from build123d import *

# Parameters (mm, degrees)
SKETCH1_R           = 6
BOSS_EXTRUDE1_DEPTH = 6


with BuildPart() as part:
    # Sketch1 → Boss-Extrude1 (new body, symmetric)
    with BuildSketch(Plane(origin=(0, 0, 0), x_dir=(1, 0, 0), z_dir=(0, 1, 0))):
        Polygon((15.011106999, 0), (7.505553499, 13), (-7.505553499, 13), (-15.011106999, 0), (-7.505553499, -13), (7.505553499, -13), align=None)
        Circle(SKETCH1_R, mode=Mode.SUBTRACT)
    extrude(amount=BOSS_EXTRUDE1_DEPTH, both=True)

    # Sketch3 → Cut-Revolve1 (revolve, cut)
    with BuildSketch(Plane.XY):
        with BuildLine():
            Line((10.011106999, 6), (15.011106999, 6))
            Line((15.011106999, 6), (15.011106999, 1))
            ThreePointArc((15.011106999, 1), (13.546640905, 4.535533906), (10.011106999, 6))
        make_face()
    cut_revolve1 = revolve(axis=Axis((0, 1.164773658, 0), (0, 1, 0)), mode=Mode.SUBTRACT)

    # Mirror1: Cut-Revolve1 across plane
    add(cut_revolve1.mirror(Plane.ZX), mode=Mode.SUBTRACT)


solid = part.part
Geometry: final body of the model. Coordinates: model frame, mm. Round coordinates to 2 decimals unless told otherwise and drop trailing zeros. Loops run counter-clockwise (first coordinate to the right, second up) from the corner with the lowest first, then second, coordinate; pieces in that order, holes last.
Q1. Material intervals for L1, parallel to Z at x = 0, y = -1; L2, parallel to X at y = 1.25, z = 0; L3, parallel to Z at x = -3.5, y = -2, sorted ascending.
Q2. Section A-A on x = 0. Return loops of the section in (y, z).
Q3. Section B-B on y = -3.75. Return loops of the section in (x, z), plus the area to 3 significant figures.
Q4. Section C-C on y = 2.5. Return loops of the section in (x, z).
Q5. Pin query (flat end, axial travel): P1, Ø4, axis at y = 4, z = -9.5, coming from the +X side; P2, Ø1.5, axis at x = 9.5, y = 1.5, coming from the -Z side. Return the tip coordinate at first contact, or that it passes through.
Q6. Pull-direction query (X, two-part tool) for faces 1 (the cylindrical face through (-6, 0, 0)), 2 (the flat face through (11.2, 0.1, 6.6)), 3 (the flat face through (-11.2, 0.1, -6.6)), 4 (the flat face through (0, 0, 13)); classes: released by +X, released by -X, zero draft, split by the parting line, or undercut.
Evaluation:
1. L1: z = -13 to -6, 6 to 13
1. L2: x = -15 to -6, 6 to 15
1. L3: z = -13 to -4.87, 4.87 to 13
2. outline: (-6, -10.01) arc R5 ccw to (-5.01, -13) - (5.01, -13) arc R5 ccw to (6, -10.01) - (6, -6) - (-6, -6) - close; (-6, 6) - (6, 6) - (6, 10.01) arc R5 ccw to (5.01, 13) - (-5.01, 13) arc R5 ccw to (-6, 10.01) - close
3. outline: (-14.1, -1.58) - (-8.42, -11.42) arc R14.19 ccw to (-5.68, -13) - (5.68, -13) arc R14.19 ccw to (8.42, -11.42) - (14.1, -1.58) arc R14.19 ccw to (14.1, 1.58) - (8.42, 11.42) arc R14.19 ccw to (5.68, 13) - (-5.68, 13) arc R14.19 ccw to (-8.42, 11.42) - (-14.1, 1.58) arc R14.19 ccw to start; hole circle Ø12 at (0, 0)
3. area: 465 mm2
4. outline: (-14.78, -0.41) - (-7.74, -12.59) arc R14.78 ccw to (-7.03, -13) - (7.03, -13) arc R14.78 ccw to (7.74, -12.59) - (14.78, -0.41) arc R14.78 ccw to (14.78, 0.41) - (7.74, 12.59) arc R14.78 ccw to (7.03, 13) - (-7.03, 13) arc R14.78 ccw to (-7.74, 12.59) - (-14.78, 0.41) arc R14.78 ccw to start; hole circle Ø12 at (0, 0)
5. P1: stops at x = 10.68
5. P2: stops at z = -10.84
6. face 1: undercut
6. face 2: released by +X
6. face 3: released by -X
6. face 4: zero draft
